Here's how the part is built. I have some questions about the finished solid (model axes, mm). A direction names the side the tool comes from. Give positions to 0.01 mm unless a question says otherwise; leave off trailing zeros. Write each loop counter-clockwise with the first axis right and the second up, starting at its lowest first coordinate (ties: lowest second). Pieces come first, ordered by that corner, then holes. Notation, with made-up numbers: (80, -21) -> (123, -21) arc R19 cw to (123, 9) -> close; hole circle Ø1 at (-29.75, -29). An arc over 180 degrees is marked (long way). Answer as CSV lines item,"result". Start each with the question number.
from build123d import *

# Parameters (mm, degrees)
F1_R      = 4
F1_R_2    = 8.5
F2_DEPTH  = 2
F4_DEPTH  = 6
F5_R      = 0.8
F6_DEPTH  = 4.618034
F8_DEPTH  = 8
F9_R      = 1.4
F10_DEPTH = 10
F11_R     = 2
F12_DEPTH = 3
F13_W     = 9.5
F13_H     = 9.5
F13_R     = 4
F14_DEPTH = 1
F15_R     = 0.9
F16_DEPTH = 5
F18_DEPTH = 0.2


with BuildPart() as f2:
    # F1 (on Front) → F2 (new body)
    with BuildSketch(Plane.XZ):
        Polygon((-22, 25.5), (-22, 0.118034), (-19.690983, -4.5), (19.690983, -4.5), (22, 0.118034), (22, 25.5), align=None)
        with Locations((-12.3, 13)):
            Circle(F1_R, mode=Mode.SUBTRACT)
        with Locations((10.94, 11.55)):
            Circle(F1_R_2, mode=Mode.SUBTRACT)
    extrude(amount=F2_DEPTH)

    # F3 (on face) → F4 (join)
    with BuildSketch(Plane(origin=(0, 0, 0), x_dir=(-1, 0, 0), z_dir=(0, 1, 0))):
        Polygon((22, 0.118034), (-22, 0.118034), (-19.690983, -4.5), (19.690983, -4.5), align=None)
    extrude(amount=F4_DEPTH)

    # F5 (on face) → F6 (cut, through all)
    with BuildSketch(Plane(origin=(0, 0, -4.5), x_dir=(1, 0, 0), z_dir=(0, 0, -1))):
        with Locations((-17, -1)):
            Circle(F5_R)
        with Locations((17, -1)):
            Circle(F5_R)
    extrude(amount=-F6_DEPTH, mode=Mode.SUBTRACT)

    # F7 (on face) → F8 (join)
    with BuildSketch(Plane(origin=(0, 0, 0), x_dir=(-1, 0, 0), z_dir=(0, 1, 0))):
        with BuildLine():
            ThreePointArc((-17.408219, 17.06472), (-15.997514, 18.381658), (-14.326099, 19.346431))
            ThreePointArc((-14.326099, 19.346431), (-19.025005, 22.471173), (-17.408219, 17.06472))
        make_face()
        with BuildLine():
            ThreePointArc((-4.471781, 6.03528), (-5.882486, 4.718342), (-7.553901, 3.753569))
            ThreePointArc((-7.553901, 3.753569), (-7.618397, 3.399372), (-7.64, 3.04))
            Line((-7.64, 3.04), (-7.64, 0.118034))
            Line((-7.64, 0.118034), (-2.4, 0.118034))
            Line((-2.4, 0.118034), (-2.4, 5.035595))
            ThreePointArc((-2.4, 5.035595), (-3.336266, 5.741903), (-4.471781, 6.03528))
        make_face()
    extrude(amount=F8_DEPTH)

    # F9 (on face) → F10 (cut, through all)
    with BuildSketch(Plane(origin=(0, 8, 0), x_dir=(-1, 0, 0), z_dir=(0, 1, 0))):
        with Locations((-17.24, 20.06)):
            Circle(F9_R)
        with Locations((-4.64, 3.04)):
            Circle(F9_R)
    extrude(amount=-F10_DEPTH, mode=Mode.SUBTRACT)

    # F11 (on face) → F12 (join)
    with BuildSketch(Plane(origin=(0, 0, 0), x_dir=(-1, 0, 0), z_dir=(0, 1, 0))):
        with Locations((-0.1, 23.5)):
            Circle(F11_R)
        with Locations((12.4, 23.5)):
            Circle(F11_R)
        with BuildLine():
            Line((1.9, 0.118034), (1.9, 2.5))
            ThreePointArc((1.9, 2.5), (1.144335, 4.065768), (-0.55163, 4.44834))
            ThreePointArc((-0.55163, 4.44834), (-1.556353, 4.488475), (-2.4, 5.035595))
            Line((-2.4, 5.035595), (-2.4, 0.118034))
            Line((-2.4, 0.118034), (1.9, 0.118034))
        make_face()
        with BuildLine():
            Line((14.4, 0.118034), (14.4, 2.5))
            ThreePointArc((14.4, 2.5), (12.4, 4.5), (10.4, 2.5))
            Line((10.4, 2.5), (10.4, 0.118034))
            Line((10.4, 0.118034), (14.4, 0.118034))
        make_face()
    extrude(amount=F12_DEPTH)

    # F13 (on face) → F14 (cut)
    with BuildSketch(Plane(origin=(0, 0, 0), x_dir=(-1, 0, 0), z_dir=(0, 1, 0))):
        with Locations((12.3, 13)):
            Rectangle(F13_W, F13_H)
        with Locations((12.3, 13)):
            Circle(F13_R, mode=Mode.SUBTRACT)
    extrude(amount=-F14_DEPTH, mode=Mode.SUBTRACT)

    # F15 (on face) → F16 (cut, through all)
    with BuildSketch(Plane(origin=(0, 3, 0), x_dir=(-1, 0, 0), z_dir=(0, 1, 0))):
        with Locations((-0.1, 23.5)):
            Circle(F15_R)
        with Locations((12.4, 23.5)):
            Circle(F15_R)
        with Locations((-0.1, 2.5)):
            Circle(F15_R)
        with Locations((12.4, 2.5)):
            Circle(F15_R)
    extrude(amount=-F16_DEPTH, mode=Mode.SUBTRACT)

    # F17 (on face) → F18 (join)
    with BuildSketch(Plane.XZ.offset(2)):
        with BuildLine():
            ThreePointArc((-22, 28.5), (-24.12132, 27.62132), (-25, 25.5))
            Line((-25, 25.5), (-25, 0.118034))
            ThreePointArc((-25, 0.118034), (-24.919747, -0.571225), (-24.683282, -1.223607))
            Line((-24.683282, -1.223607), (-22.374265, -5.841641))
            ThreePointArc((-22.374265, -5.841641), (-21.268176, -7.051952), (-19.690983, -7.5))
            Line((-19.690983, -7.5), (19.690983, -7.5))
            ThreePointArc((19.690983, -7.5), (21.268176, -7.051952), (22.374265, -5.841641))
            Line((22.374265, -5.841641), (24.683282, -1.223607))
            ThreePointArc((24.683282, -1.223607), (24.919747, -0.571225), (25, 0.118034))
            Line((25, 0.118034), (25, 25.5))
            ThreePointArc((25, 25.5), (24.12132, 27.62132), (22, 28.5))
            Line((22, 28.5), (-22, 28.5))
        make_face()
        Polygon((-22, 0.118034), (-22, 25.5), (22, 25.5), (22, 0.118034), (19.690983, -4.5), (-19.690983, -4.5), align=None, mode=Mode.SUBTRACT)
    extrude(amount=-F18_DEPTH)


solid = f2.part
Item 1: If I drill on line 1 (Z direction, x = -12.4, y = 0.2); line 2 (Z direction, x = 0.1, y = -0.05); line 3 (Z direction, x = -12.3, y = -1.4), over which ranges is the centre line in solid material (lowest first)? Write a range as [from, to].
Item 2: If we section it at C-C (y = -0.5): State how many separate pieces and enclosed holes the cut face has, and give its area (3 significant figures).
Item 3: I'm going to push flat-ended pins straight in: pin 1 (3.5 mm diameter, centred on x = 17.24, z = 20.06, fed in from -Y); pin 2 (4 mm diameter, centred on y = 4.5, z = 3.5, fed in from -X); pin 3 (1.3 mm diameter, centred on x = 0, z = 3, fed in from +Y); pin 4 (6 mm diameter, centred on x = -16.5, y = 3.5, fed in from +Z). Where does each tip first touch, or does it pass through?
Item 4: If we section it at A-A (y = 4.75): Please give me the cut outline in (x, z), and give its area (3 significant figures).
Item 5: For faces 1 (the face through (-1.9, 1, 1)), 2 (the face through (-14.4, 1, 1)), 3 (the face through (-12.2, -0.5, 17.75)), 4 (the face through (15, 3, 0.118)), which set-ups out of +Z, -Z, +X, -X, +Y, -Y let a thin tool reach every point of the face, with its end or its side?
Item 6: If we section it at B-B (x = 10.94): Please give me the cut outline in (y, z).
Item 7: We'd pull the mould along Z, two halves only. Please class faces 5 (the face through (-12.2, -0.5, 8.25)), 6 (the face through (20.86, 2.05, -2.16)), 7 (the face through (-22, -1, 13)), 8 (the face through (3.321, 3.944, 5.735)): released by +Z, released by -Z, zero draft, split by the parting line, or undercut.
Item 8: If we section it at D-D (z = 14): Please give me the cut outline in (x, y), and give its area (3 significant figures).
Final values:
1,line 1,"[-4.5, 1.6], [3.4, 4.5], [21.5, 22.6], [24.4, 25.5]"
1,line 2,"[-4.5, 1.6], [3.4, 22.6], [24.4, 25.5]"
1,line 3,"[-4.5, 1.61], [3.39, 9], [17, 22.61], [24.39, 25.5]"
2,separate pieces,"1"
2,enclosed holes,"8"
2,area,"970 mm2"
3,pin 1,"y = -2"
3,pin 2,"x = -14.4"
3,pin 3,"y = 3"
3,pin 4,"z = 25.14"
4,outline,"(-22, 0.12) -> (-19.69, -4.5) -> (19.69, -4.5) -> (22, 0.12) -> (7.64, 0.12) -> (7.64, 3.04) arc R3 ccw to (7.55, 3.75) arc R8.5 cw to (4.47, 6.04) arc R3 ccw to (2.4, 5.04) -> (2.4, 0.12) -> close; (14.33, 19.35) arc R8.5 cw to (17.41, 17.06) arc R3 ccw (long way) to start; hole circle Ø2.8 at (4.64, 3.04); hole circle Ø2.8 at (17.24, 20.06)"
4,area,"232 mm2"
5,face 1,"+Z, +Y"
5,face 2,"+Z, -X, +Y"
5,face 3,"+Y"
5,face 4,"+X, +Y"
6,outline,"(-2, -7.5) -> (-1.8, -7.5) -> (-1.8, -4.5) -> (6, -4.5) -> (6, 0.12) -> (0, 0.12) -> (0, 3.05) -> (-2, 3.05) -> close; (-2, 20.05) -> (0, 20.05) -> (0, 25.5) -> (-1.8, 25.5) -> (-1.8, 28.5) -> (-2, 28.5) -> close"
7,face 5,"undercut"
7,face 6,"released by -Z"
7,face 7,"zero draft"
7,face 8,"released by +Z"
8,outline,"(-25, -2) -> (-16.17, -2) -> (-16.17, -1) -> (-17.05, -1) -> (-17.05, 0) -> (-22, 0) -> (-22, -1.8) -> (-25, -1.8) -> close; (-8.43, -2) -> (2.8, -2) -> (2.8, 0) -> (-7.55, 0) -> (-7.55, -1) -> (-8.43, -1) -> close; (19.08, -2) -> (25, -2) -> (25, -1.8) -> (22, -1.8) -> (22, 0) -> (19.08, 0) -> close"
8,area,"39.4 mm2"
